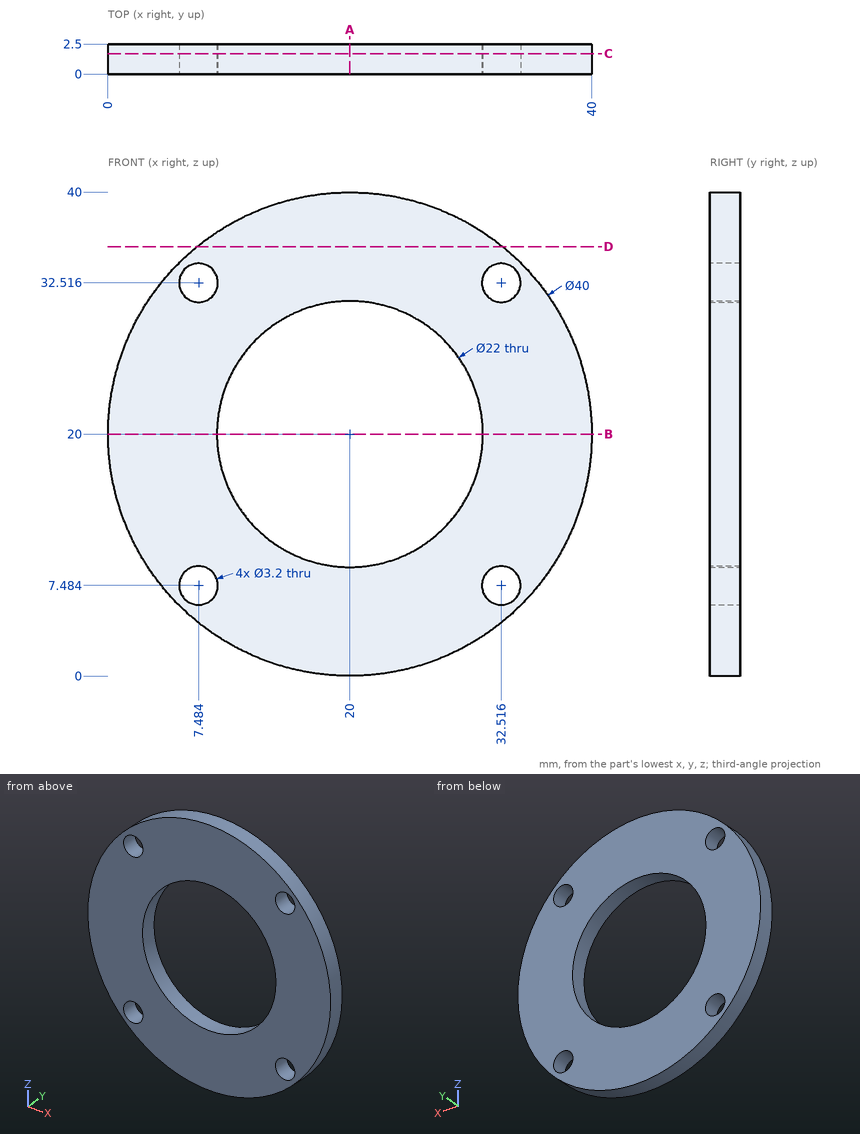
Input: dimensioned drawing with shaded views. Units: mm. Origin: part minimum x, y, z. Round coordinates to 2 decimals unless told otherwise and drop trailing zeros. Order: outer loops, then holes, each group sorted by start corner. A loop starts at its lowest first (then second) coordinate and runs counter-clockwise, first axis right, second up. Notation, with made-up numbers: (41, -3) -> (68, -3) arc R31 ccw to (68, 35) -> close; hole circle Ø11 at (88, -23.5). An arc over 180 degrees is marked (long way). Put each result on its own line as item: value. Start each with the question number.
Q1. Section D-D on z = 35.5. Return the cut outline in (x, y), and give its area (3 significant figures).
Q2. Section B-B on z = 20. Return the cut outline in (x, y), and give its area (3 significant figures).
Q3. Section C-C on y = 1.7. Return the cut outline in (x, z).
Q4. Line query: probe 1 along X at (y, z) = (1.85, 20); probe 2 along Z at (x, y) = (7, 1.65); probe 3 along X at (y, z) = (1.6, 7.5) (1 decimal). Output: solid intervals per line, ascending.
Q5. Section A-A on x = 20. Return the cut outline in (y, z).
Q6. First-contact query: pin 1 (1.5 mm diameter, centred on y = 1, z = 11, fed in from -X). Flat tip, straight axial feed; report the tip coordinate or a pass-through.
Ans:
1. outline: (7.36, 0) -> (32.64, 0) -> (32.64, 2.5) -> (7.36, 2.5) -> close
1. area: 63.2 mm2
2. outline: (0, 0) -> (9, 0) -> (9, 2.5) -> (0, 2.5) -> close; (31, 0) -> (40, 0) -> (40, 2.5) -> (31, 2.5) -> close
2. area: 45.0 mm2
3. outline: circle Ø40 at (20, 20); hole circle Ø3.2 at (7.48, 7.48); hole circle Ø3.2 at (7.48, 32.52); hole circle Ø22 at (20, 20); hole circle Ø3.2 at (32.52, 7.48); hole circle Ø3.2 at (32.52, 32.52)
4. probe 1: x = 0 to 9, 31 to 40
4. probe 2: z = 4.8 to 5.96, 9.01 to 30.99, 34.04 to 35.2
4. probe 3: x = 4.4 to 5.9, 9.1 to 30.9, 34.1 to 35.6
5. outline: (0, 0) -> (2.5, 0) -> (2.5, 9) -> (0, 9) -> close; (0, 31) -> (2.5, 31) -> (2.5, 40) -> (0, 40) -> close
6. pin 1: stops at x = 1.78
